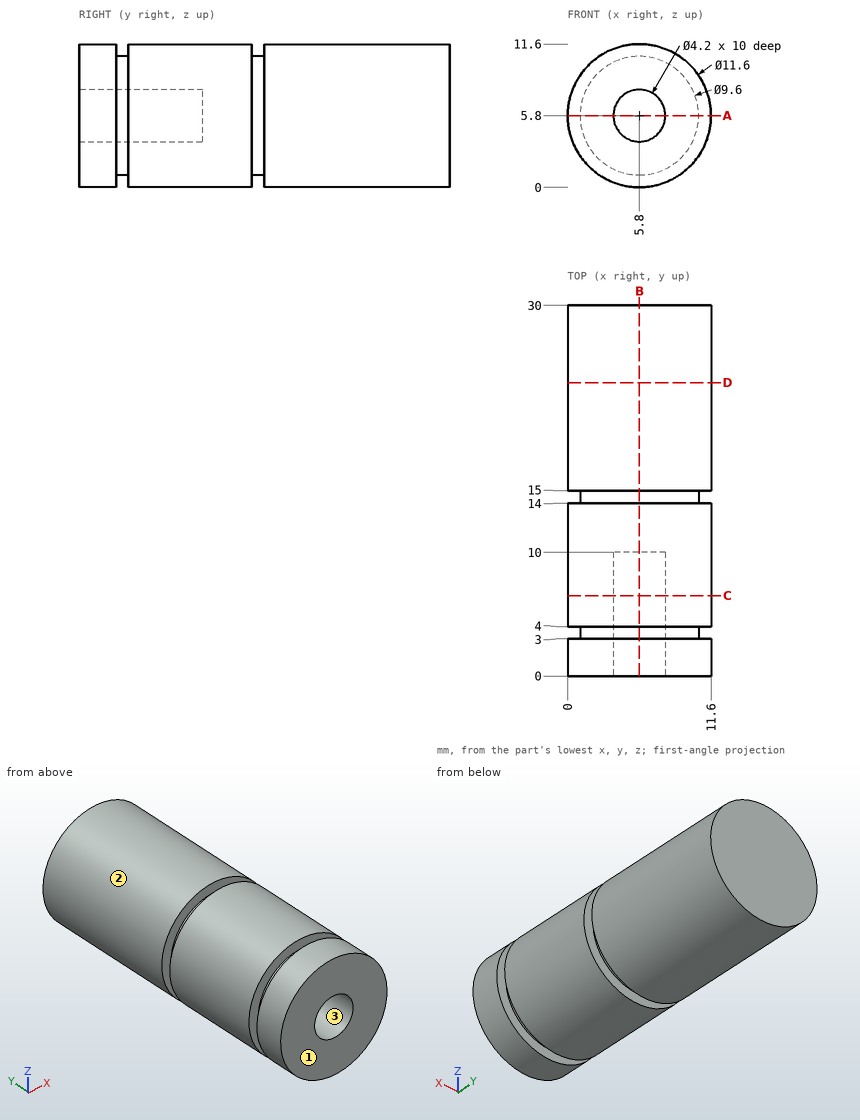
Geometry check sheet. Reference: drawing and pictorial views, mm from the part's lowest x, y, z. Give positions to 0.01 mm unless a question says otherwise; leave off trailing zeros. Write each loop counter-clockwise with the first axis right and the second up, starting at its lowest first coordinate (ties: lowest second). Pieces come first, ordered by that corner, then holes. Notation, with made-up numbers: M 84,-19 L 135,-19 A25 ccw 135,11 Z; hole C -31.5,-3.5 d7. An arc over 180 degrees is marked long. Put each result on its own line as item: value. Start each with the question number.
1. Scan lines: line 1 along Y through (x, z) = (8.25, 10); line 2 along X through (y, z) = (2.75, 5.8); line 3 along Y through (x, z) = (6.5, 5.25). Record each from-to range of solid material in increasing order. Write a range as [from, to].
2. Draft check along X on the marked faces 1, 2 and 3. Enter one of: +X half, -X half, draft (parallel to the pull), parting line (faces both ways), or undercut.
3. Section check A-A (z = 5.8). Record the cut outline in (x, y).
4. Go/stop test with flat-tipped pins: pin 1 Ø5 at (x, y) = (9.5, 13) entering from +Z; pin 2 Ø5 at (x, y) = (8.5, 21) entering from -Z; pin 3 Ø1.5 at (y, z) = (11.5, 4) entering from +X. Record where each tip stops, or that it passes through.
5. Section check C-C (y = 6.5). Record the cut outline in (x, z), and give its area (3 significant figures).
6. Section check D-D (y = 23.75). Record the cut outline in (x, z), and give its area (3 significant figures).
7. Section check B-B (x = 5.8). Record the cut outline in (y, z).
Answer list:
1. line 1: [0, 3], [4, 14], [15, 30]
1. line 2: [0, 3.7], [7.9, 11.6]
1. line 3: [10, 30]
2. face 1: draft
2. face 2: parting line
2. face 3: undercut
3. outline: M 0,0 L 3.7,0 L 3.7,10 L 7.9,10 L 7.9,0 L 11.6,0 L 11.6,3 L 10.6,3 L 10.6,4 L 11.6,4 L 11.6,14 L 10.6,14 L 10.6,15 L 11.6,15 L 11.6,30 L 0,30 L 0,15 L 1,15 L 1,14 L 0,14 L 0,4 L 1,4 L 1,3 L 0,3 Z
4. pin 1: z = 11.47
4. pin 2: z = 0
4. pin 3: x = 11.5
5. outline: C 5.8,5.8 d11.6; hole C 5.8,5.8 d4.2
5. area: 91.8 mm2
6. outline: C 5.8,5.8 d11.6
6. area: 106 mm2
7. outline: M 0,0 L 3,0 L 3,1 L 4,1 L 4,0 L 14,0 L 14,1 L 15,1 L 15,0 L 30,0 L 30,11.6 L 15,11.6 L 15,10.6 L 14,10.6 L 14,11.6 L 4,11.6 L 4,10.6 L 3,10.6 L 3,11.6 L 0,11.6 L 0,7.9 L 10,7.9 L 10,3.7 L 0,3.7 Z
